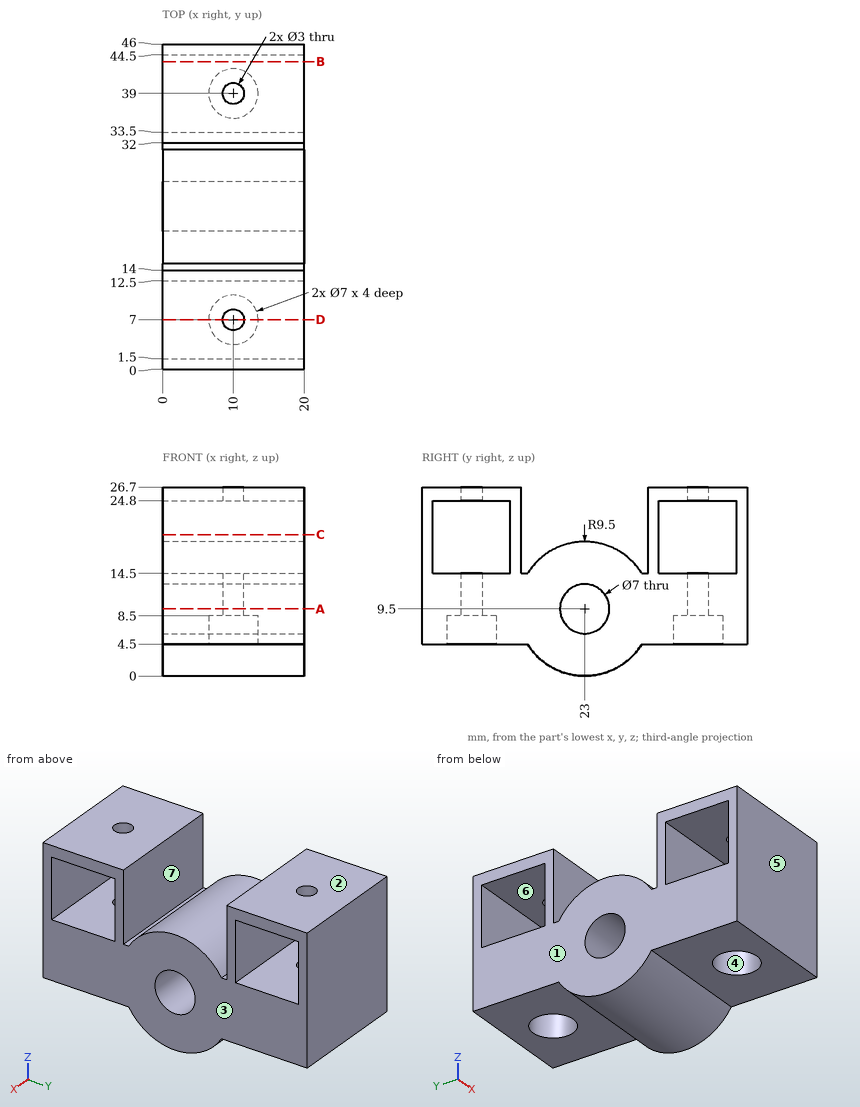
The figure shows three views and two pictorial views of one solid part (mm, origin at its lowest corner). Answer the questions. A direction names the side the tool comes from. Round coordinates to 2 decimals unless told otherwise and drop trailing zeros. Write each loop counter-clockwise with the first axis right and the second up, starting at its lowest first coordinate (ties: lowest second). Pieces come first, ordered by that corner, then holes. Notation, with made-up numbers: (38, -12) - (79, -12) arc R20 cw to (79, 23) - close; hole circle Ø3 at (-23, 0.5). An arc over 180 degrees is marked (long way). Answer in a Markdown table with one row per item. Add a question column.
1. A cutting plane is placed at B-B, the plane y = 43.5. Determine the outline of the cut face in (x, z).
2. A cutting plane is placed at A-A, the plane z = 9.5. Determine the outline of the cut face in (x, y).
3. The mould has two halves that part along X. Classify the marked faces 1, 2, 3 and 4: +X half, -X half, draft (parallel to the pull), parting line (faces both ways), or undercut.
4. A cutting plane is placed at C-C, the plane z = 20. Determine the outline of the cut face in (x, y).
5. For the marked faces 5, 6 and 7, determine the directions among +Z, -Z, +X, -X, +Y, -Y from which every point of the face is accessible in a straight line to the end or side of a thin tool.
6. Find the intervals of material crossed by line 1 along Y through (x, z) = (10, 26.05); line 2 along Y through (x, z) = (2, 22.75); line 3 along Y through (x, z) = (10, 5.55), in increasing order. Write a range as from..to.
7. Given pin 1 (2 mm diameter, centred on x = 9, y = 37.5, fed in from -Z); pin 2 (2 mm diameter, centred on x = 10, y = 7, fed in from -Z); pin 3 (12 mm diameter, centred on x = 12.5, y = 36, fed in from -Z); pin 4 (5 mm diameter, centred on x = 6.5, y = 14.5, fed in from -Z), each flat-ended and moving along its own axis, determine where each tip first touches the part or whether it passes through.
8. A cutting plane is placed at D-D, the plane y = 7. Determine the outline of the cut face in (x, z), and give its area (3 significant figures).
Worked out:
| question | item | result |
|---|---|---|
| 1 | outline | (0, 4.5) - (20, 4.5) - (20, 14.5) - (0, 14.5) - close; (0, 24.8) - (20, 24.8) - (20, 26.7) - (0, 26.7) - close |
| 2 | outline | (0, 0) - (20, 0) - (20, 19.5) - (0, 19.5) - close; (0, 26.5) - (20, 26.5) - (20, 46) - (0, 46) - close; hole circle Ø3 at (10, 7); hole circle Ø3 at (10, 39) |
| 3 | face 1 | -X half |
| 3 | face 2 | draft |
| 3 | face 3 | +X half |
| 3 | face 4 | undercut |
| 4 | outline | (0, 0) - (20, 0) - (20, 1.5) - (0, 1.5) - close; (0, 12.5) - (20, 12.5) - (20, 14) - (0, 14) - close; (0, 32) - (20, 32) - (20, 33.5) - (0, 33.5) - close; (0, 44.5) - (20, 44.5) - (20, 46) - (0, 46) - close |
| 5 | face 5 | +Z, -Z, +X, -X, -Y |
| 5 | face 6 | +X, -X |
| 5 | face 7 | +Z, +X, -X |
| 6 | line 1 | 0..5.5, 8.5..14, 32..37.5, 40.5..46 |
| 6 | line 2 | 0..1.5, 12.5..14, 32..33.5, 44.5..46 |
| 6 | line 3 | 0..3.5, 10.5..35.5, 42.5..46 |
| 7 | pin 1 | z = 8.5 |
| 7 | pin 2 | through |
| 7 | pin 3 | z = 3.08 |
| 7 | pin 4 | z = 2.13 |
| 8 | outline | (0, 4.5) - (6.5, 4.5) - (6.5, 8.5) - (8.5, 8.5) - (8.5, 14.5) - (0, 14.5) - close; (0, 24.8) - (8.5, 24.8) - (8.5, 26.7) - (0, 26.7) - close; (11.5, 8.5) - (13.5, 8.5) - (13.5, 4.5) - (20, 4.5) - (20, 14.5) - (11.5, 14.5) - close; (11.5, 24.8) - (20, 24.8) - (20, 26.7) - (11.5, 26.7) - close |
| 8 | area | 186 mm^2 |
